from build123d import *

# Parameters (mm, degrees)
SKETCH1_R               = 60
SKETCH1_R_2             = 2
BOSS_EXTRUDE1_DEPTH     = 10
SKETCH2_R               = 10.05
SKETCH2_R_2             = 5.05
BOSS_EXTRUDE2_DEPTH     = 20
CUT_EXTRUDE1_DEPTH      = 20
CUT_EXTRUDE1_DEPTH_BACK = 20
SKETCH3_R               = 1.75


with BuildPart() as part:
    # Sketch1 → Boss-Extrude1 (new body)
    with BuildSketch(Plane.XY):
        Circle(SKETCH1_R)
        with Locations((-15.5, 15.5)):
            Circle(SKETCH1_R_2, mode=Mode.SUBTRACT)
        with Locations((15.5, 15.5)):
            Circle(SKETCH1_R_2, mode=Mode.SUBTRACT)
        with Locations((15.5, -15.5)):
            Circle(SKETCH1_R_2, mode=Mode.SUBTRACT)
        with Locations((-15.5, -15.5)):
            Circle(SKETCH1_R_2, mode=Mode.SUBTRACT)
    extrude(amount=BOSS_EXTRUDE1_DEPTH)

    # Sketch2 → Boss-Extrude2 (add)
    # profile 1 of 2: a face of its own
    with BuildSketch(Plane.XY.offset(10)):
        Circle(SKETCH2_R)
        Circle(SKETCH2_R_2, mode=Mode.SUBTRACT)
    # profile 2 of 2: a face of its own
    with BuildSketch(Plane.XY.offset(10)):
        with BuildLine():
            ThreePointArc((3.016620626, 4.05), (0, 5.05), (-3.016620626, 4.05))
            Line((-3.016620626, 4.05), (0, 4.05))
            Line((0, 4.05), (3.016620626, 4.05))
        make_face()
    extrude(amount=BOSS_EXTRUDE2_DEPTH)

    # Sketch3 → Cut-Extrude1 (cut, two sides: drawn at the far end of the back side and taken through both)
    with BuildSketch(Plane(origin=(0, 4.05, 0), x_dir=(-1, 0, 0), z_dir=(0, -1, 0)).offset(-CUT_EXTRUDE1_DEPTH_BACK)):
        with Locations(Location((0, -20, 0), (0, 0, 270))):
            Circle(SKETCH3_R)
    extrude(amount=CUT_EXTRUDE1_DEPTH + CUT_EXTRUDE1_DEPTH_BACK, mode=Mode.SUBTRACT)


solid = part.part
Could you check a few things on this model? Use its own coordinates, in mm. A direction names the side the tool comes from. Coordinates: 2 decimals unless noted, no trailing zeros. Loops run counter-clockwise (first coordinate to the right, second up) from the corner with the lowest first, then second, coordinate; pieces in that order, holes last.
1. Imagine slicing it at A-A (z = 20). Please give me the cut outline in (x, y).
2. Imagine slicing it at D-D (y = 15.5). Please give me the cut outline in (x, z), and give its area (3 significant figures).
3. For P1, Ø4, axis at x = 0, z = 20, coming from the -Y side; P2, Ø3, axis at x = -44, y = 32.5, coming from the +Z side; P3, Ø3, axis at x = 25.5, z = 12, coming from the +Y side; P4, Ø2, axis at y = -31, z = 8.5, coming from the +X side, each with a flat end and sliding along its axis, tell me the tip position at first contact or that it passes through.
4. For faces 1 (the face through (15.24, -13.517, 4.93)), 2 (the face through (-2.813, -4.194, 19.86)), which set-ups out of +Z, -Z, +X, -X, +Y, -Y let a thin tool reach every point of the face, with its end or its side?
5. Imagine slicing it at B-B (x = 0). Please give me the cut outline in (y, z), and give its area (3 significant figures).
6. Imagine slicing it at C-C (y = 0). Please give me the cut outline in (x, z).
7. I need wall thicknesses on L1, parallel to Y at x = -15, z = 4; L2, parallel to Y at x = 0, z = 15.75. Which ranges of each line are inside material? Lowest first, please.
8. We'd pull the mould along Z, two halves only. Please class faces 3 (the face through (-1, 1, 0)), 4 (the face through (12, 1, 10)), 5 (the face through (-0.08, -7.36, 18.25)): released by +Z, released by -Z, zero draft, split by the parting line, or undercut.
Computed values:
1. outline: (-3.02, 4.05) - (-1.75, 4.05) - (-1.75, 9.9) arc R10.05 ccw to (-1.75, -9.9) - (-1.75, -4.74) arc R5.05 cw to start; (1.75, -9.9) arc R10.05 ccw to (1.75, 9.9) - (1.75, 4.05) - (3.02, 4.05) arc R5.05 cw to (1.75, -4.74) - close
2. outline: (-57.96, 0) - (-17.5, 0) - (-17.5, 10) - (-57.96, 10) - close; (-13.5, 0) - (13.5, 0) - (13.5, 10) - (-13.5, 10) - close; (17.5, 0) - (57.96, 0) - (57.96, 10) - (17.5, 10) - close
2. area: 1,080 mm2
3. P1: stops at y = -10.05
3. P2: stops at z = 10
3. P3: passes through
3. P4: stops at x = 51.96
4. face 1: +Z, -Z
4. face 2: +Z
5. outline: (-60, 0) - (60, 0) - (60, 10) - (10.05, 10) - (10.05, 18.25) - (4.05, 18.25) - (4.05, 10) - (-5.05, 10) - (-5.05, 18.25) - (-10.05, 18.25) - (-10.05, 10) - (-60, 10) - close; (-10.05, 21.75) - (-5.05, 21.75) - (-5.05, 30) - (-10.05, 30) - close; (4.05, 21.75) - (10.05, 21.75) - (10.05, 30) - (4.05, 30) - close
5. area: 1,380 mm2
6. outline: (-60, 0) - (60, 0) - (60, 10) - (10.05, 10) - (10.05, 30) - (5.05, 30) - (5.05, 10) - (-5.05, 10) - (-5.05, 30) - (-10.05, 30) - (-10.05, 10) - (-60, 10) - close
7. L1: y = -58.09 to -17.44, -13.56 to 13.56, 17.44 to 58.09
7. L2: y = -10.05 to -5.05, 4.05 to 10.05
8. face 3: released by -Z
8. face 4: released by +Z
8. face 5: undercut
